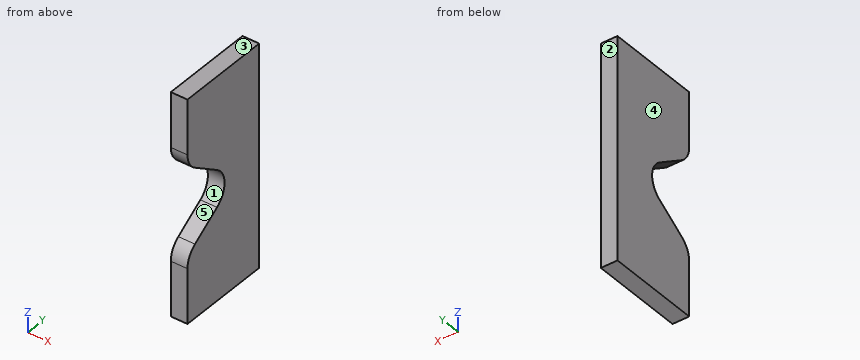
from build123d import *

# Parameters (mm, degrees)
BOSS_EXTRUDE1_DEPTH = 19.05


with BuildPart() as part:
    # Sketch1 → Boss-Extrude1 (new body)
    with BuildSketch(Plane(origin=(0, 0, 0), x_dir=(0, 0, -1), z_dir=(1, 0, 0))):
        with BuildLine():
            Line((-127, 0), (-127, 107.95))
            Line((-127, 107.95), (127, 107.95))
            Line((127, 107.95), (127, 0))
            Line((127, 0), (64.393667466, 0))
            ThreePointArc((64.393667466, 0), (52.408476157, 3.005465191), (43.259589989, 11.310615016))
            Line((43.259589989, 11.310615016), (21.134077476, 44.498883786))
            ThreePointArc((21.134077476, 44.498883786), (0, 55.809498802), (-21.134077476, 44.498883786))
            Line((-21.134077476, 44.498883786), (-43.259589989, 11.310615016))
            ThreePointArc((-43.259589989, 11.310615016), (-52.408476157, 3.005465191), (-64.393667466, 0))
            Line((-64.393667466, 0), (-127, 0))
        make_face()
    extrude(amount=BOSS_EXTRUDE1_DEPTH)


solid = part.part
Verification items for the finished model (mm, model axes). Face numbers are marked on the shaded views. A direction names the side the tool comes from. Give positions to 0.01 mm unless a question says otherwise; leave off trailing zeros. Write each loop counter-clockwise with the first axis right and the second up, starting at its lowest first coordinate (ties: lowest second). Pieces come first, ordered by that corner, then holes. Notation, with made-up numbers: (0.5, 14.5) - (15.5, 14.5) arc R30 ccw to (15.5, 51.5) - close; hole circle Ø7 at (39, 83). An arc over 180 degrees is marked (long way). Answer as CSV lines item,"result". Start each with the question number.
1. Sectioned sample at D-D (z = 25). Record the boundary of the cut face in (x, y), then the cut area to 3 significant figures.
2. Sectioned sample at A-A (x = 12.5). Record the boundary of the cut face in (y, z), then the cut area to 3 significant figures.
3. Set-up check for the marked faces 4 and 5: record each of +Z, -Z, +X, -X, +Y, -Y from which the full face is reachable in a straight line by a thin tool's end or side.
4. Draft check along Z on the marked faces 1, 2 and 3. Enter one of: pulls with the +Z half, pulls with the -Z half, needs draft (parallel to the pull), parting line crosses it, or undercut.
5. Depth check by flat-ended pin: pin 1 (6 mm diameter, centred on x = 9.5, z = 14.5, fed in from -Y). Enter the tip coordinate at first touch or a pass-through.
6. Thickness scan on line 1 (Y direction, x = 9, z = 63.5); line 2 (Z direction, x = 14, y = 21); line 3 (Z direction, x = 6, y = 15). Record the ranges inside material, lowest first.
7. Sectioned sample at B-B (y = 37). Record the boundary of the cut face in (x, z), then the cut area to 3 significant figures.
8. Sectioned sample at C-C (z = -32.5). Record the boundary of the cut face in (x, y), then the cut area to 3 significant figures.
Derived:
1,outline,"(0, 38.7) - (19.05, 38.7) - (19.05, 107.95) - (0, 107.95) - close"
1,area,"1,320 mm²"
2,outline,"(0, -127) - (107.95, -127) - (107.95, 127) - (0, 127) - (0, 64.39) arc R25.4 ccw to (11.31, 43.26) - (44.5, 21.13) arc R25.4 cw to (44.5, -21.13) - (11.31, -43.26) arc R25.4 ccw to (0, -64.39) - close"
2,area,"23,800 mm²"
3,face 4,"+Z, -Z, -X, +Y, -Y"
3,face 5,"+X, -X, -Y"
4,face 1,"undercut"
4,face 2,"needs draft"
4,face 3,"pulls with the +Z half"
5,pin 1,"y = 48.82"
6,line 1,"0.02 to 107.95"
6,line 2,"-127 to -36.8, 36.8 to 127"
6,line 3,"-127 to -40.8, 40.8 to 127"
7,outline,"(0, -127) - (19.05, -127) - (19.05, -26.13) - (0, -26.13) - close; (0, 26.13) - (19.05, 26.13) - (19.05, 127) - (0, 127) - close"
7,area,"3,840 mm²"
8,outline,"(0, 27.45) - (19.05, 27.45) - (19.05, 107.95) - (0, 107.95) - close"
8,area,"1,530 mm²"
